Geometry check sheet. Reference: the model listing, model coordinates, mm. A direction names the side the tool comes from. Round coordinates to 2 decimals unless told otherwise and drop trailing zeros. Loops run counter-clockwise (first coordinate to the right, second up) from the corner with the lowest first, then second, coordinate; pieces in that order, holes last. Notation, with made-up numbers: M -22,36.5 L 35,36.5 A21 cw 35,61.5 Z; hole C -0.75,18 d1. An arc over 180 degrees is marked long. Answer in a Markdown table with one row per item. Add a question column.
```python
from build123d import *

# Parameters (mm, degrees)
SKETCH1_W                        = 8.5
SKETCH1_H                        = 12
BOSS_EXTRUDE1_DEPTH              = 41.5
CUT_EXTRUDE1_DEPTH               = 43.784342931
M1_6_HOLE1_FIXINGPCB_D           = 1.8
M1_6_HOLE1_FIXINGPCB_CSINK_D     = 3.6
M1_6_HOLE1_FIXINGPCB_CSINK_ANGLE = 90
FILLET1_R                        = 0.5
M1_6_HOLE2_INTUNION_D            = 1.8
M1_6_HOLE2_INTUNION_DEPTH        = 200
M1_6_HOLE2_INTUNION_TIP          = 0.540774557
M1_6_HOLE3_EXTUNION_D            = 1.8
M1_6_HOLE3_EXTUNION_DEPTH        = 3
M1_6_HOLE3_EXTUNION_TIP          = 0.540774557
M1_6_HOLE4_TOPUNION_D            = 1.8
M1_6_HOLE4_TOPUNION_DEPTH        = 3
M1_6_HOLE4_TOPUNION_TIP          = 0.540774557
M1_6_CLEARANCE_HOLE1_D           = 1.8
M1_6_CLEARANCE_HOLE1_DEPTH       = 3
M1_6_CLEARANCE_HOLE1_TIP         = 0.540774557


with BuildPart() as part:
    # Sketch1 → Boss-Extrude1 (new, symmetric)
    with BuildSketch(Plane.XY):
        Rectangle(SKETCH1_W, SKETCH1_H)
    extrude(amount=BOSS_EXTRUDE1_DEPTH, both=True)

    # Sketch2 → Cut-Extrude1 (cut, through all)
    with BuildSketch(Plane(origin=(4.25, 0, 0), x_dir=(0, 0, -1), z_dir=(1, 0, 0))):
        with BuildLine():
            Line((-37.5, 1), (37.5, 1))
            ThreePointArc((37.5, 1), (38.207106781, 0.707106781), (38.5, 0))
            Line((38.5, 0), (38.5, -6))
            Line((38.5, -6), (-38.5, -6))
            Line((-38.5, -6), (-38.5, 0))
            ThreePointArc((-38.5, 0), (-38.207106781, 0.707106781), (-37.5, 1))
        make_face()
    extrude(amount=-CUT_EXTRUDE1_DEPTH, mode=Mode.SUBTRACT)

    # M1.6 Hole1-FixingPCB (through all)
    with Locations(Plane.ZY.offset(4.25)):
        with Locations((-21.5, 3.5), (21.5, 3.5)):
            CounterSinkHole(M1_6_HOLE1_FIXINGPCB_D / 2, M1_6_HOLE1_FIXINGPCB_CSINK_D / 2, counter_sink_angle=M1_6_HOLE1_FIXINGPCB_CSINK_ANGLE)

    # Fillet1
    fillet1_edges = [part.edges().sort_by_distance(p)[0] for p in [
        (0, -6, 41.5),
        (0, -6, -38.5),
        (0, -6, 38.5),
        (0, -6, -41.5),
        (0, 6, -41.5),
        (0, 6, 41.5),
    ]]
    fillet(fillet1_edges, radius=FILLET1_R)

    # M1.6 Hole2-IntUnion
    with Locations(Plane.XY.offset(41.5)):
        with Locations((0, -3)):
            Hole(M1_6_HOLE2_INTUNION_D / 2, depth=M1_6_HOLE2_INTUNION_DEPTH)
            with Locations((0, 0, -(M1_6_HOLE2_INTUNION_DEPTH + M1_6_HOLE2_INTUNION_TIP / 2))):  # 118° drill point
                Cone(0, M1_6_HOLE2_INTUNION_D / 2, M1_6_HOLE2_INTUNION_TIP, mode=Mode.SUBTRACT)

    # M1.6 Hole3-ExtUnion
    with Locations(Plane.ZY.offset(4.25)):
        with Locations((-35.5, 3.5), (35.5, 3.5)):
            Hole(M1_6_HOLE3_EXTUNION_D / 2, depth=M1_6_HOLE3_EXTUNION_DEPTH)
            with Locations((0, 0, -(M1_6_HOLE3_EXTUNION_DEPTH + M1_6_HOLE3_EXTUNION_TIP / 2))):  # 118° drill point
                Cone(0, M1_6_HOLE3_EXTUNION_D / 2, M1_6_HOLE3_EXTUNION_TIP, mode=Mode.SUBTRACT)

    # M1.6 Hole4-TopUnion
    with Locations(Plane(origin=(4.25, 0, 0), x_dir=(0, 0, -1), z_dir=(1, 0, 0))):
        with Locations((0, 3.5)):
            Hole(M1_6_HOLE4_TOPUNION_D / 2, depth=M1_6_HOLE4_TOPUNION_DEPTH)
            with Locations((0, 0, -(M1_6_HOLE4_TOPUNION_DEPTH + M1_6_HOLE4_TOPUNION_TIP / 2))):  # 118° drill point
                Cone(0, M1_6_HOLE4_TOPUNION_D / 2, M1_6_HOLE4_TOPUNION_TIP, mode=Mode.SUBTRACT)

    # M1.6 Clearance Hole1
    with Locations(Plane(origin=(0, 6, 0), x_dir=(1, 0, 0), z_dir=(0, 1, 0))):
        with Locations((0, 29), (0, -29)):
            Hole(M1_6_CLEARANCE_HOLE1_D / 2, depth=M1_6_CLEARANCE_HOLE1_DEPTH)
            with Locations((0, 0, -(M1_6_CLEARANCE_HOLE1_DEPTH + M1_6_CLEARANCE_HOLE1_TIP / 2))):  # 118° drill point
                Cone(0, M1_6_CLEARANCE_HOLE1_D / 2, M1_6_CLEARANCE_HOLE1_TIP, mode=Mode.SUBTRACT)


solid = part.part
```
1) Cross-section at A-A, the plane z = 21.5. Record the boundary of the cut face in (x, y), plus the area to 3 significant figures.
2) Set-up check for faces 1 (the cylindrical face through (0.195, 4.479, 29.879)), 2 (the cylindrical face through (-2.73, 2.95, 36.21)), 3 (the flat face through (1, -2, -38.5)): record each of +Z, -Z, +X, -X, +Y, -Y from which the full face is reachable in a straight line by a thin tool's end or side.
3) Go/stop test with flat-tipped pins: pin 1 (6 mm diameter, centred on y = -1.5, z = 16, fed in from -X); pin 2 (2.5 mm diameter, centred on x = 0, z = 15.5, fed in from -Y); pin 3 (1.4 mm diameter, centred on y = 3.5, z = 21.5, fed in from -X). Record where each tip stops, or that it passes through.
4) Draft check along Z on faces 4 (the flat face through (0, 0, 41.5)), 5 (the flat face through (0, 1, 1)), 6 (the cylindrical face through (0.195, -3.879, -40.021)). Enter one of: +Z half, -Z half, draft (parallel to the pull), parting line (faces both ways), or undercut.
5) Thickness scan on L1, parallel to Z at x = -2.2, y = 3.5; L2, parallel to X at y = 4.5, z = -29; L3, parallel to Z at x = -0.75, y = -4.5. Record the ranges inside material, lowest first. Write a range as [from, to].
Worked answers:
| question | item | result |
|---|---|---|
| 1 | outline | M -4.25,1 L 4.25,1 L 4.25,2.6 L -3.35,2.6 L -4.25,1.7 Z; M -4.25,5.3 L -3.35,4.4 L 4.25,4.4 L 4.25,6 L -4.25,6 Z |
| 1 | area | 26.4 mm2 |
| 2 | face 1 | +Y |
| 2 | face 2 | -X |
| 2 | face 3 | +X, -X, -Y |
| 3 | pin 1 | stops at x = -4.25 |
| 3 | pin 2 | stops at y = 1 |
| 3 | pin 3 | passes through |
| 4 | face 4 | +Z half |
| 4 | face 5 | undercut |
| 4 | face 6 | draft |
| 5 | L1 | z = [-41.5, -36.4], [-34.6, -22.4], [-20.6, 20.6], [22.4, 34.6], [36.4, 41.5] |
| 5 | L2 | x = [-4.25, -0.9], [0.9, 4.25] |
| 5 | L3 | z = [-41.5, -38.5], [38.5, 41.5] |
